For this review, use the dimensioned drawing (mm, ordinates from the lowest corner) and the shaded views. A direction names the side the tool comes from. Round coordinates to 2 decimals unless told otherwise and drop trailing zeros. Loops run counter-clockwise (first coordinate to the right, second up) from the corner with the lowest first, then second, coordinate; pieces in that order, holes last. Notation, with made-up numbers: M -6.5,26.25 L 28.5,26.25 A12 cw 28.5,31.25 Z; hole C 21.5,-2.75 d11. An arc over 180 degrees is marked long. Use a Markdown table: item, result. Add a question column.
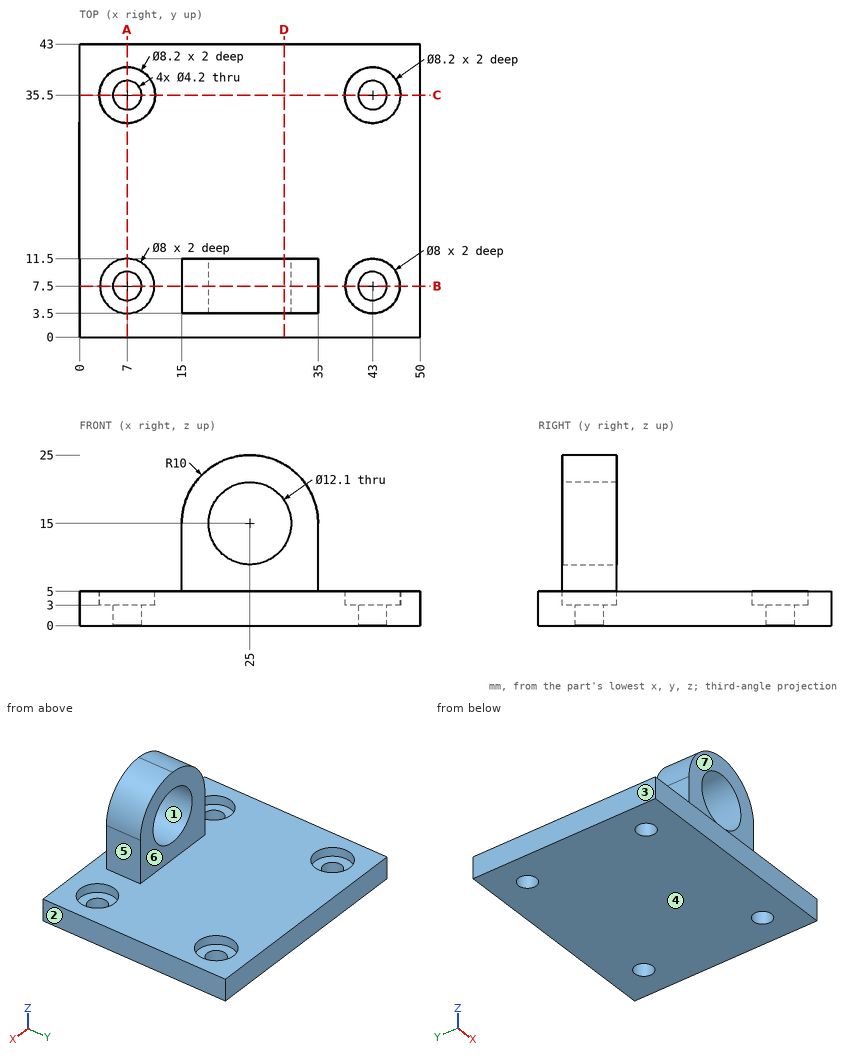
(1) For the marked faces 4, 5, 6 and 7, list the 3-axis set-ups (+Z, -Z, +X, -X, +Y, -Y) from which the entire face can be reached by the end or side of a thin tool; tool diameter is ignored.
(2) Consider section B-B, the plane y = 7.5. Give the boundary of the cut face in (x, z), then the cut area to 3 significant figures.
(3) Draft analysis for pull direction X (two halves, no side actions). For the marked faces 1, 2 and 3, state which applies: released by +X, released by -X, zero draft, split by the parting line, or undercut.
(4) Consider section C-C, the plane y = 35.5. Give the boundary of the cut face in (x, z).
(5) Consider section A-A, the plane x = 7. Give the boundary of the cut face in (y, z), then the cut area to 3 significant figures.
(6) Insertion check: pin 1 Ø10 at (x, z) = (26.5, 10.5) entering from +Y; pin 2 Ø1 at (x, y) = (10.5, 28) entering from +Z; pin 3 Ø4 at (x, y) = (42, 7.5) entering from +Z. Each pin has a flat end and moves straight along its axis. Give the tip position at first contact, or say it passes through.
(7) To check wall thickness, follow probe 1 along Y at (x, z) = (43, 1.2); probe 2 along Y at (x, z) = (7, 3.9); probe 3 along X at (y, z) = (7.5, 1.85). State the ranges of each line that lie inside material, in increasing order.
(8) Consider section D-D, the plane x = 30. Give the boundary of the cut face in (y, z), then the cut area to 3 significant figures.
Found:
| question | item | result |
|---|---|---|
| 1 | face 4 | -Z, +X, -X, +Y, -Y |
| 1 | face 5 | +Z, +X, +Y, -Y |
| 1 | face 6 | +Z, +X, -X, +Y |
| 1 | face 7 | +Z, +X, -X, -Y |
| 2 | outline | M 0,0 L 4.9,0 L 4.9,3 L 3,3 L 3,5 L 0,5 Z; M 9.1,0 L 40.9,0 L 40.9,3 L 39,3 L 39,5 L 35,5 L 35,15 A10 ccw 15,15 L 15,5 L 11,5 L 11,3 L 9.1,3 Z; M 45.1,0 L 50,0 L 50,5 L 47,5 L 47,3 L 45.1,3 Z; hole C 25,15 d12.1 |
| 2 | area | 435 mm^2 |
| 3 | face 1 | undercut |
| 3 | face 2 | released by +X |
| 3 | face 3 | released by -X |
| 4 | outline | M 0,0 L 4.9,0 L 4.9,3 L 2.9,3 L 2.9,5 L 0,5 Z; M 9.1,0 L 40.9,0 L 40.9,3 L 38.9,3 L 38.9,5 L 11.1,5 L 11.1,3 L 9.1,3 Z; M 45.1,0 L 50,0 L 50,5 L 47.1,5 L 47.1,3 L 45.1,3 Z |
| 5 | outline | M 0,0 L 5.4,0 L 5.4,3 L 3.5,3 L 3.5,5 L 0,5 Z; M 9.6,0 L 33.4,0 L 33.4,3 L 31.4,3 L 31.4,5 L 11.5,5 L 11.5,3 L 9.6,3 Z; M 37.6,0 L 43,0 L 43,5 L 39.6,5 L 39.6,3 L 37.6,3 Z |
| 5 | area | 157 mm^2 |
| 6 | pin 1 | stops at y = 11.5 |
| 6 | pin 2 | stops at z = 5 |
| 6 | pin 3 | stops at z = 3 |
| 7 | probe 1 | y = 0 to 5.4, 9.6 to 33.4, 37.6 to 43 |
| 7 | probe 2 | y = 0 to 3.5, 11.5 to 31.4, 39.6 to 43 |
| 7 | probe 3 | x = 0 to 4.9, 9.1 to 40.9, 45.1 to 50 |
| 8 | outline | M 0,0 L 43,0 L 43,5 L 11.5,5 L 11.5,11.59 L 3.5,11.59 L 3.5,5 L 0,5 Z; M 3.5,18.41 L 11.5,18.41 L 11.5,23.66 L 3.5,23.66 Z |
| 8 | area | 310 mm^2 |
